Part model, mm, in its own coordinate system. Face numbers are marked on the shaded views. A direction names the side the tool comes from. Give positions to 0.01 mm unless a question says otherwise; leave off trailing zeros. Order: outer loops, then holes, each group sorted by start corner. A loop starts at its lowest first (then second) coordinate and runs counter-clockwise, first axis right, second up. Notation, with made-up numbers: (-31, 77.5) -> (4, 77.5) arc R15 cw to (4, 83.5) -> close; hole circle Ø2 at (-8.5, 6.5). An arc over 180 degrees is marked (long way). Write item = value, one per line. Start each with the question number.
(1) Two-plate mould, pull along X, no slides. Class the marked faces 1, 2, 3 and 4: pulls with the +X half, pulls with the -X half, needs draft (parallel to the pull), parting line crosses it, or undercut.
(2) Saw through at D-D, the plane x = 41. List the corners of the cut face in (y, z), then the cut area to 3 significant figures.
(3) Saw through at C-C, the plane y = 60.5. List the corners of the cut face in (x, z), then the cut area to 3 significant figures.
(4) Flat gauge pins, fed straight in: pin 1 (1 mm diameter, centred on x = 101, y = 14.5, fed in from -Z); pin 2 (3 mm diameter, centred on y = 49.5, z = 7, fed in from -X); pin 3 (9 mm diameter, centred on x = 7, y = 53.5, fed in from -Z). Where does each tip first touch, or does it go through?
(5) Saw through at A-A, the plane x = 103. List the corners of the cut face in (y, z), then the cut area to 3 significant figures.
(6) Probe line 1 along X through (y, z) = (100, 61.5); line 2 along Y through (x, z) = (144, 49.5); line 3 along Z through (x, y) = (148, 57). List the from-to ranges inside material, lowest first. Write a range as from..to.
(7) Which spindle directions (+Z, -Z, +X, -X, +Y, -Y) get a long thin tool onto all of the face, cutting with end or side? Do the marked faces 5, 6 and 7. Say none if no direction does.
(8) Saw through at B-B, the plane z = 32. List the corners of the cut face in (x, y).
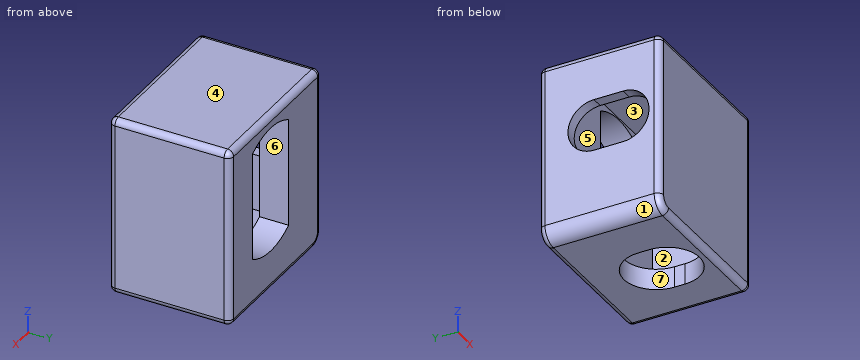
from build123d import *

# Parameters (mm, degrees)
SKETCH_W             = 160
SKETCH_H             = 119
PAD_DEPTH            = 175.5
THICKNESS_T          = -11
SKETCH001_W          = 138
SKETCH001_H          = 9.5
PAD001_DEPTH         = 108
SKETCH002_W          = 160
SKETCH002_H          = 175.5
PAD002_DEPTH         = 28.5
POCKET_DEPTH         = 20.5
POCKET001_DEPTH      = 11
POCKET002_DEPTH      = 32
POCKET002_DEPTH_BACK = 1
FILLET_R             = 14.5
FILLET001_R          = 6


with BuildPart() as part:
    # Sketch → Pad (new body)
    with BuildSketch(Plane.XY):
        with Locations((80, 59.5)):
            Rectangle(SKETCH_W, SKETCH_H)
    extrude(amount=PAD_DEPTH)

    # Thickness
    thickness_openings = [part.faces().sort_by_distance(p)[0] for p in [
        (80, 119, 87.75),
    ]]
    offset(amount=THICKNESS_T, openings=thickness_openings, kind=Kind.INTERSECTION)

    # Sketch001 (on Face6 of Thickness) → Pad001 (join)
    with BuildSketch(Plane(origin=(0, 119, 0), x_dir=(-1, 0, 0), z_dir=(0, 1, 0))):
        with Locations((-80, 15.75)):
            Rectangle(SKETCH001_W, SKETCH001_H)
    extrude(amount=-PAD001_DEPTH)

    # Sketch002 (on Face6 of Pad001) → Pad002 (join)
    with BuildSketch(Plane(origin=(0, 119, 0), x_dir=(-1, 0, 0), z_dir=(0, 1, 0))):
        with Locations((-80, 87.75)):
            Rectangle(SKETCH002_W, SKETCH002_H)
    extrude(amount=-PAD002_DEPTH)

    # Sketch003 (on Face4 of Pad002) → Pocket (cut)
    with BuildSketch(Plane(origin=(0, 0, 0), x_dir=(1, 0, 0), z_dir=(0, 0, -1))):
        with BuildLine():
            ThreePointArc((120.75, -42.749927), (88.999969, -11), (57.25, -42.749988))
            Line((57.25, -42.749988), (57.25, -53.450058))
            ThreePointArc((57.25, -53.450058), (89.000056, -85.2), (120.75, -53.449945))
            Line((120.75, -53.449945), (120.75, -42.749927))
        make_face()
    extrude(amount=-POCKET_DEPTH, mode=Mode.SUBTRACT)

    # Sketch004 (on Face2 of Pocket) → Pocket001 (cut)
    with BuildSketch(Plane(origin=(0, 0, 0), x_dir=(0, -1, 0), z_dir=(-1, 0, 0))):
        with BuildLine():
            ThreePointArc((-65, 127), (-90.5, 101.5), (-65, 76))
            Line((-65, 76), (-36.5, 76))
            ThreePointArc((-36.5, 76), (-11, 101.5), (-36.5, 127))
            Line((-65, 127), (-36.5, 127))
        make_face()
    extrude(amount=-POCKET001_DEPTH, mode=Mode.SUBTRACT)

    # Sketch005 (on Face6 of Pocket001) → Pocket002 (cut, two sides)
    with BuildSketch(Plane(origin=(0, 119, 0), x_dir=(-1, 0, 0), z_dir=(0, 1, 0))) as pocket002_sk:
        with BuildLine():
            ThreePointArc((-57.249999, 154.253521), (-88.999999, 163), (-120.749999, 154.253521))
            Line((-120.749999, 47.746479), (-120.749999, 154.253521))
            Line((-120.75, 47.746479), (-120.749999, 47.746479))
            ThreePointArc((-120.75, 47.746479), (-89, 39), (-57.249999, 47.746479))
            Line((-57.249999, 154.253521), (-57.249999, 47.746479))
        make_face()
    extrude(amount=-POCKET002_DEPTH, mode=Mode.SUBTRACT)
    extrude(pocket002_sk.sketch, amount=POCKET002_DEPTH_BACK, mode=Mode.SUBTRACT)

    # Fillet
    fillet_edges = [part.edges().sort_by_distance(p)[0] for p in [
        (0, 59.5, 0),
    ]]
    fillet(fillet_edges, radius=FILLET_R)

    # Fillet001
    fillet001_edges = [part.edges().sort_by_distance(p)[0] for p in [
        (87.25, 119, 0),
        (4.246952, 119, 4.246952),
        (0, 119, 95),
        (80, 119, 175.5),
        (160, 59.5, 175.5),
        (160, 119, 87.75),
        (160, 59.5, 0),
        (160, 0, 87.75),
        (87.25, 0, 0),
        (4.246952, 0, 4.246952),
        (0, 0, 95),
        (80, 0, 175.5),
        (0, 59.5, 175.5),
    ]]
    fillet(fillet001_edges, radius=FILLET001_R)


solid = part.part
Results list:
q1.face_1 = pulls with the -X half
q1.face_2 = undercut
q1.face_3 = undercut
q1.face_4 = needs draft
q2.outline = (0, 6) arc R6 ccw to (6, 0) -> (113, 0) arc R6 ccw to (119, 6) -> (119, 169.5) arc R6 ccw to (113, 175.5) -> (6, 175.5) arc R6 ccw to (0, 169.5) -> close; hole (11, 20.5) -> (90.5, 20.5) -> (90.5, 164.5) -> (11, 164.5) -> close
q2.area = 9,410 mm^2
q3.outline = (0, 14.5) arc R14.5 ccw to (14.5, 0) -> (58.04, 0) -> (58.04, 20.5) -> (11, 20.5) -> (11, 76) -> (0, 76) -> close; (0, 127) -> (11, 127) -> (11, 164.5) -> (149, 164.5) -> (149, 20.5) -> (119.96, 20.5) -> (119.96, 0) -> (154, 0) arc R6 ccw to (160, 6) -> (160, 169.5) arc R6 ccw to (154, 175.5) -> (6, 175.5) arc R6 ccw to (0, 169.5) -> close
q3.area = 6,310 mm^2
q4.pin_1 = 164.5
q4.pin_2 = 1.3
q4.pin_3 = 0.31
q5.outline = (0, 6) arc R6 ccw to (6, 0) -> (14.25, 0) -> (14.25, 20.5) -> (11, 20.5) -> (11, 164.5) -> (90.5, 164.5) -> (90.5, 161.4) -> (119, 161.4) -> (119, 169.5) arc R6 ccw to (113, 175.5) -> (6, 175.5) arc R6 ccw to (0, 169.5) -> close; (81.95, 0) -> (113, 0) arc R6 ccw to (119, 6) -> (119, 40.6) -> (90.5, 40.6) -> (90.5, 20.5) -> (81.95, 20.5) -> close
q5.area = 4,580 mm^2
q6.line_1 = 0..57.25, 120.75..160
q6.line_2 = 0..11, 90.5..119
q6.line_3 = 0..20.5, 164.5..175.5
q7.face_5 = none
q7.face_6 = +Y
q7.face_7 = -Z
q8.outline = (0, 6) arc R6 ccw to (6, 0) -> (154, 0) arc R6 ccw to (160, 6) -> (160, 113) arc R6 ccw to (154, 119) -> (6, 119) arc R6 ccw to (0, 113) -> close; hole (11, 11) -> (149, 11) -> (149, 90.5) -> (11, 90.5) -> close
